Answer from the drawing. Dimensions are ordinates in mm from the lowest x, y and z of the part. A direction names the side the tool comes from. Coordinates: 2 decimals unless noted, no trailing zeros. Order: outer loops, then holes, each group sorted by start corner. A loop starts at its lowest first (then second) coordinate and runs counter-clockwise, first axis right, second up. Notation, with made-up numbers: (69, 60.5) - (83, 60.5) arc R19 cw to (83, 74.5) - close; hole circle Ø2 at (13, 32.25). An arc over 180 degrees is marked (long way). Answer as a JSON object with one key per item and string values. Group by question number.
1) The mould has two halves that part along X. Classify the marked faces 3, 4 and 5: released by +X, released by -X, zero draft, split by the parting line, or undercut.
2) Section B-B (y = 60.5) is taken. Give the vertices of the cut face in (x, z).
3) This flat-tipped pin is pushed along its axis until it touches: P1, Ø2.5, axis at x = 5, y = 95, coming from the -Z side. Where does it stop, or does it pass through?
4) Section D-D (y = 80) is taken. Give the vertices of the cut face in (x, z).
5) Find the intervals of material crossed by line 1 along X through (y, z) = (95, 1.2); line 2 along Z through (x, y) = (15.25, 72.5); line 3 along Y through (x, z) = (25, 1), in increasing order.
6) A tool of negligible diameter and unlimited length cuts with its end or side. For the marked faces 1 and 2, from which of +Z, -Z, +X, -X, +Y, -Y can it reach the whole face along a straight path? Write none if from no direction.
7) Section A-A (x = 5) is taken. Count the separate pieces of the cut face and the enclosed holes in it, plus the area to 3 significant figures.
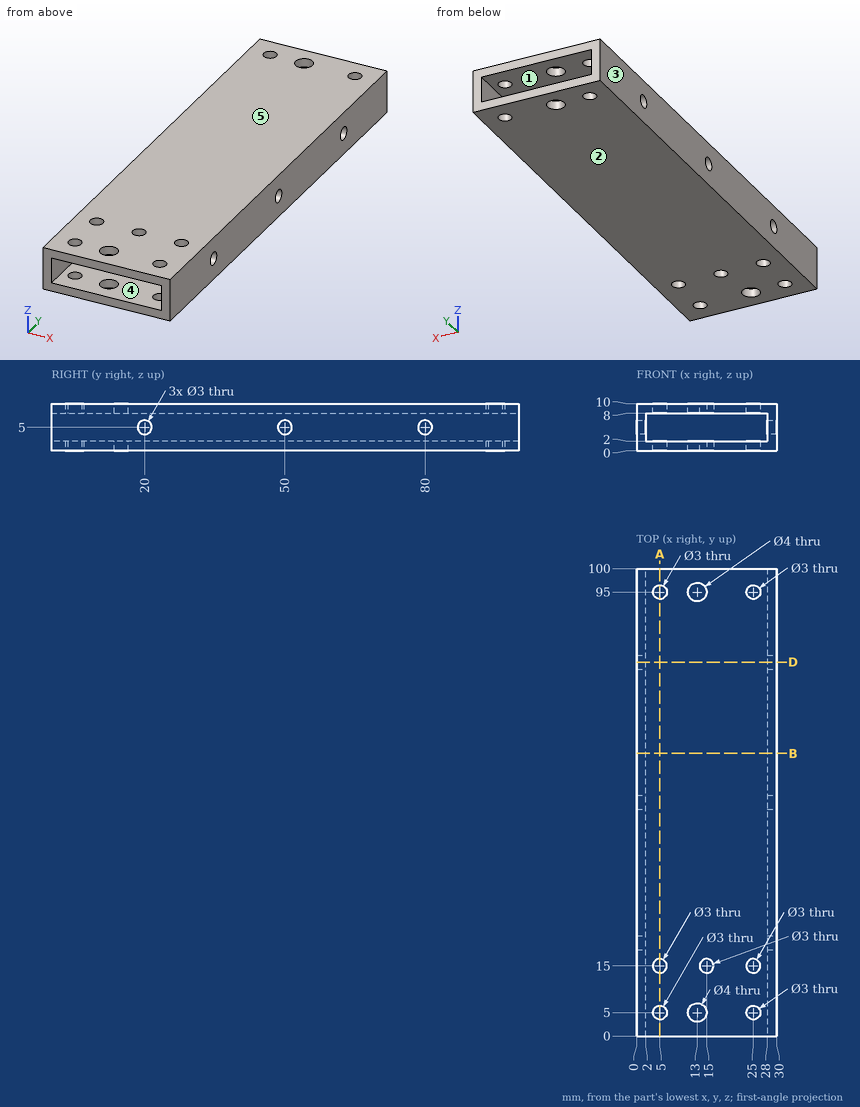
Report:
{
 "1": {"face 3": "released by -X", "face 4": "undercut", "face 5": "zero draft"},
 "2": {"outline": "(0, 0) - (30, 0) - (30, 10) - (0, 10) - close; hole (2, 2) - (28, 2) - (28, 8) - (2, 8) - close"},
 "3": {"P1": "passes through"},
 "4": {"outline": "(0, 0) - (30, 0) - (30, 3.5) - (28, 3.5) - (28, 2) - (2, 2) - (2, 3.5) - (0, 3.5) - close; (0, 6.5) - (2, 6.5) - (2, 8) - (28, 8) - (28, 6.5) - (30, 6.5) - (30, 10) - (0, 10) - close"},
 "5": {"line 1": "x = 0 to 3.5, 6.5 to 11, 15 to 23.5, 26.5 to 30", "line 2": "z = 0 to 2, 8 to 10", "line 3": "y = 0 to 3.5, 6.5 to 13.5, 16.5 to 93.5, 96.5 to 100"},
 "6": {"face 1": "+Y, -Y", "face 2": "-Z, +X, -X, +Y, -Y"},
 "7": {"separate pieces": "8", "enclosed holes": "0", "area": "364 mm²"}
}
